The model under review builds one solid part; all positions refer to its coordinate system, in mm. Face numbers are marked on the shaded views. A direction names the side the tool comes from. Coordinates: 2 decimals unless noted, no trailing zeros. Loops run counter-clockwise (first coordinate to the right, second up) from the corner with the lowest first, then second, coordinate; pieces in that order, holes last. Notation, with made-up numbers: (14.25, -10) - (18.25, -10) arc R30 ccw to (18.25, 25) - close; hole circle Ø4 at (37.25, 47). An arc over 180 degrees is marked (long way). One line per item, written item: value. Start each with the question number.
1. For the marked faces 5, 6 and 7, list the 3-axis set-ups (+Z, -Z, +X, -X, +Y, -Y) from which the entire face can be reached by the end or side of a thin tool; tool diameter is ignored.
2. We need section A-A, the plane z = 2.5. Give the boundary of the cut face in (x, y).
3. To check wall thickness, follow line 1 (X direction, y = 0.95, z = 2); line 2 (Z direction, x = -5.5, y = 2.3); line 3 (X direction, y = 2.25, z = -2.75). State the ranges of each line that lie inside material, in increasing order.
4. Insertion check: P1, Ø1, axis at x = -6.5, y = 1.5, coming from the +Z side; P2, Ø1.5, axis at x = -7, z = -4.5, coming from the -Y side; P3, Ø0.8, axis at x = -4.5, y = 1.5, coming from the +Z side; P4, Ø1.2, axis at y = 1, z = 3, coming from the +X side. Each pin has a flat end and moves straight along its axis. Give the tip position at first contact, or say it passes through.
5. We need section D-D, the plane z = 8.25. Give the boundary of the cut face in (x, y), then the cut area to 3 significant figures.
6. We need section C-C, the plane y = 0.85. Give the boundary of the cut face in (x, z).
7. Mouldability with a two-part tool opening along X and no side actions: class the marked faces 1, 2, 3 and 4 as +X half, -X half, draft (parallel to the pull), parting line (faces both ways), or undercut.
8. We need section B-B, the plane z = -5.5. Give the boundary of the cut face in (x, y).
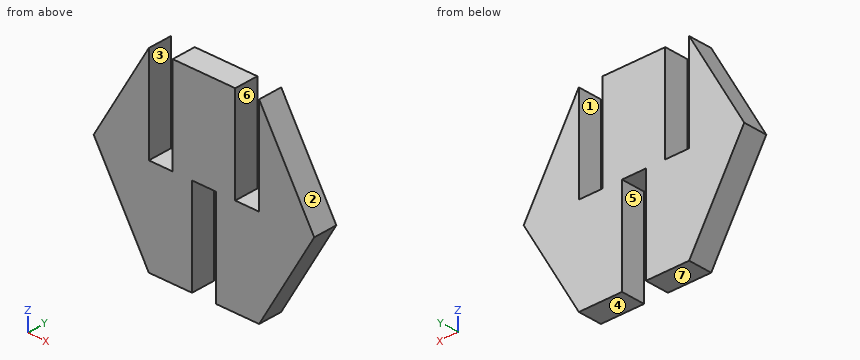
from build123d import *

# Parameters (mm, degrees)
BOSS_EXTRUDE1_DEPTH = 2.5
SKETCH5_W           = 2.5
SKETCH5_H           = 2.5
CUT_EXTRUDE3_DEPTH  = 10
SKETCH6_W           = 2.5
SKETCH6_H           = 2.5
CUT_EXTRUDE4_DEPTH  = 10
SKETCH7_W           = 2.5
SKETCH7_H           = 2.5
CUT_EXTRUDE5_DEPTH  = 10


with BuildPart() as part:
    # Sketch1 → Boss-Extrude1 (new body)
    with BuildSketch(Plane(origin=(0, 0, 0), x_dir=(1, 0, 0), z_dir=(0, 1, 0))):
        Polygon((11.547005384, 0), (5.773502692, 10), (-5.773502692, 10), (-11.547005384, 0), (-5.773502692, -10), (5.773502692, -10), align=None)
    extrude(amount=BOSS_EXTRUDE1_DEPTH)

    # Sketch5 → Cut-Extrude3 (cut)
    with BuildSketch(Plane.XY.offset(10)):
        with Locations((-4.523502692, 1.25)):
            Rectangle(SKETCH5_W, SKETCH5_H)
    extrude(amount=-CUT_EXTRUDE3_DEPTH, mode=Mode.SUBTRACT)

    # Sketch6 → Cut-Extrude4 (cut)
    with BuildSketch(Plane.XY.offset(10)):
        with Locations((4.523502692, 1.25)):
            Rectangle(SKETCH6_W, SKETCH6_H)
    extrude(amount=-CUT_EXTRUDE4_DEPTH, mode=Mode.SUBTRACT)

    # Sketch7 → Cut-Extrude5 (cut)
    with BuildSketch(Plane(origin=(0, 0, -10), x_dir=(-1, 0, 0), z_dir=(0, 0, -1))):
        with Locations((-0.001497308, 1.25)):
            Rectangle(SKETCH7_W, SKETCH7_H)
    extrude(amount=-CUT_EXTRUDE5_DEPTH, mode=Mode.SUBTRACT)


solid = part.part
Findings below:
1. face 5: -Z, +Y, -Y
1. face 6: +Z, +Y, -Y
1. face 7: -Z, +X, -X, +Y, -Y
2. outline: (-10.1, 0) - (-5.77, 0) - (-5.77, 2.5) - (-10.1, 2.5) - close; (-3.27, 0) - (3.27, 0) - (3.27, 2.5) - (-3.27, 2.5) - close; (5.77, 0) - (10.1, 0) - (10.1, 2.5) - (5.77, 2.5) - close
3. line 1: -10.39 to -5.77, -3.27 to 3.27, 5.77 to 10.39
3. line 2: -10 to 0
3. line 3: -9.96 to -1.25, 1.25 to 9.96
4. P1: z = 9.61
4. P2: y = 0
4. P3: z = 0
4. P4: x = 10.16
5. outline: (-6.78, 0) - (-5.77, 0) - (-5.77, 2.5) - (-6.78, 2.5) - close; (-3.27, 0) - (3.27, 0) - (3.27, 2.5) - (-3.27, 2.5) - close; (5.77, 0) - (6.78, 0) - (6.78, 2.5) - (5.77, 2.5) - close
5. area: 21.4 mm2
6. outline: (-11.55, 0) - (-5.77, -10) - (-1.25, -10) - (-1.25, 0) - (1.25, 0) - (1.25, -10) - (5.77, -10) - (11.55, 0) - (5.77, 10) - (5.77, 0) - (3.27, 0) - (3.27, 10) - (-3.27, 10) - (-3.27, 0) - (-5.77, 0) - (-5.77, 10) - close
7. face 1: undercut
7. face 2: +X half
7. face 3: undercut
7. face 4: draft
8. outline: (-8.37, 0) - (-1.25, 0) - (-1.25, 2.5) - (-8.37, 2.5) - close; (1.25, 0) - (8.37, 0) - (8.37, 2.5) - (1.25, 2.5) - close
